Study the drawing (mm; zero at the part's minimum x, y, z) and answer. A direction names the side the tool comes from. Coordinates: 2 decimals unless noted, no trailing zeros. Loops run counter-clockwise (first coordinate to the right, second up) from the corner with the lowest first, then second, coordinate; pieces in that order, holes last. Notation, with made-up numbers: M 62.5,86.5 L 112.5,86.5 A30 ccw 112.5,122.5 Z; hole C 78,74.5 d1. An arc over 180 degrees is marked long. Use one line per item in the form item = value. Start each with the question number.
1. The part is cut by section B-B (y = 10.5). Give the vertices of the cut face in (x, z) (1 decimal).
2. The part is cut by section C-C (x = 19). Give the vertices of the cut face in (y, z).
3. Flat-ended cylindrical pins translate along their axes: pin 1 (1 mm diameter, centred on y = 7.5, z = 9, fed in from +X) (1 decimal); pin 2 (6 mm diameter, centred on y = 22, z = 14, fed in from -X); pin 3 (3 mm diameter, centred on x = 16, z = 7.5, fed in from -Y). Find the tip coordinate at first contact, or state that the pin passes through.
4. The part is cut by section D-D (y = 36.5). Give the vertices of the cut face in (x, z), plus the area to 3 significant figures.
5. Find the intervals of material crossed by probe 1 along X at (y, z) = (4, 23.5) (1 decimal); probe 2 along X at (y, z) = (4.5, 2.25) (1 decimal); probe 3 along Y at (x, z) = (36, 6.5), in increasing order. Write a range as [from, to].
6. The part is cut by section A-A (z = 15.5). Give the vertices of the cut face in (x, y), plus the area to 3 significant figures.
7. For a pull along X with two mould halves and no side action, classify the marked faces 1, 2 and 3 as released by +X, released by -X, zero draft, split by the parting line, or undercut.
8. A tool of negligible diameter and unlimited length cuts with its end or side. For the marked faces 4 and 5, from which of +Z, -Z, +X, -X, +Y, -Y can it reach the whole face along a straight path? Write none if from no direction.
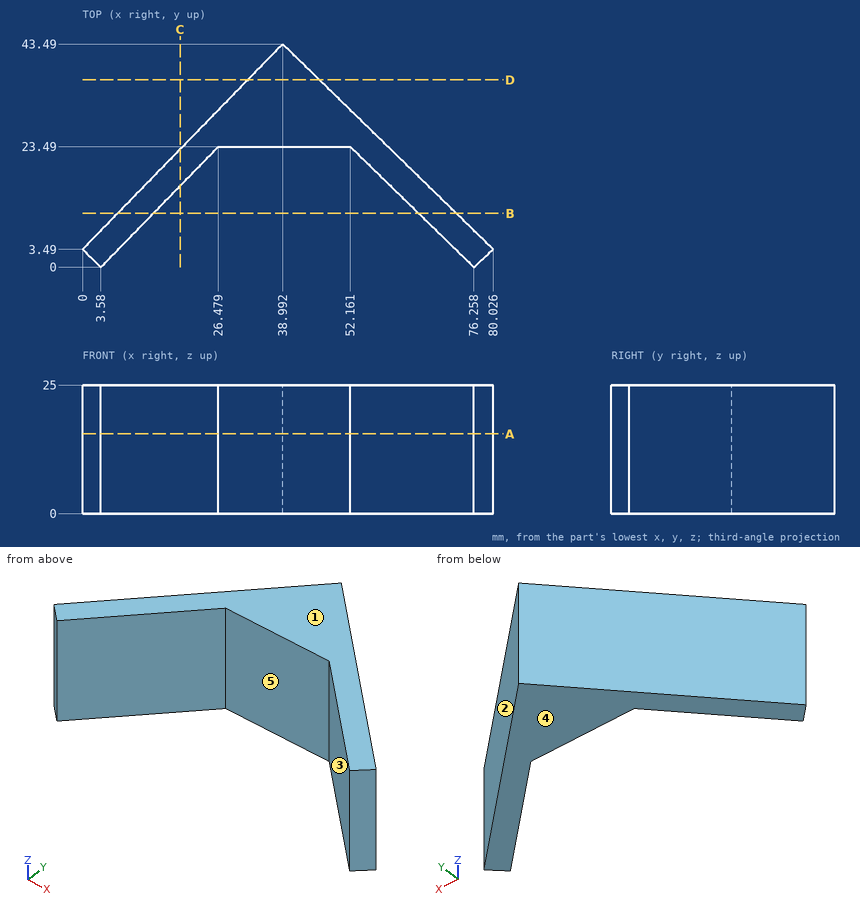
Computed values:
q1.outline = M 6.8,0 L 13.8,0 L 13.8,25 L 6.8,25 Z; M 65.5,0 L 72.8,0 L 72.8,25 L 65.5,25 Z
q2.outline = M 15.82,0 L 22.98,0 L 22.98,25 L 15.82,25 Z
q3.pin_1 = 76.4
q3.pin_2 = 15.12
q3.pin_3 = 11.2
q4.outline = M 32.18,0 L 46.16,0 L 46.16,25 L 32.18,25 Z
q4.area = 350 mm²
q5.probe_1 = [0.5, 7.5], [72.2, 79.5]
q5.probe_2 = [1, 8], [71.6, 79]
q5.probe_3 = [23.49, 40.42]
q6.outline = M 0,3.49 L 3.58,0 L 26.48,23.49 L 52.16,23.49 L 76.26,0 L 80.03,3.49 L 38.99,43.49 Z
q6.area = 712 mm²
q7.face_1 = zero draft
q7.face_2 = released by +X
q7.face_3 = undercut
q8.face_4 = -Z, +X, -X, +Y, -Y
q8.face_5 = +Z, -Z, -Y
